The listing builds one solid part. Answer for the finished solid, in the listing's coordinates (mm). A direction names the side the tool comes from. Round coordinates to 2 decimals unless told otherwise and drop trailing zeros. Answer in a Markdown table with one row per item. Add a question column.
```python
from build123d import *

# Parameters (mm, degrees)
F1_DEPTH = 7
F2_R     = 2
F3_COUNT = 3


with BuildPart() as f1:
    # F0 (on Top) → F1 (new body)
    with BuildSketch(Plane.XY):
        with BuildLine():
            ThreePointArc((28, 0), (14, 14), (0, 0))
            Line((0, 0), (3.1437343742, 0))
            Line((3.1437343742, 0), (8.3414580162, 9.3975654268))
            Line((8.3414580162, 9.3975654268), (19.3092594014, 9.5992238198))
            Line((19.3092594014, 9.5992238198), (24.9678013852, 0.201658393))
            Line((24.9678013852, 0.201658393), (24.8562656258, 0))
            Line((24.8562656258, 0), (28, 0))
        make_face()
        with BuildLine():
            Line((3.1437343742, 0), (0, 0))
            ThreePointArc((0, 0), (14, -14), (28, 0))
            Line((28, 0), (24.8562656258, 0))
            Line((24.8562656258, 0), (19.6585419838, -9.3975654268))
            Line((19.6585419838, -9.3975654268), (8.6907405986, -9.5992238198))
            Line((8.6907405986, -9.5992238198), (3.0321986148, -0.201658393))
            Line((3.0321986148, -0.201658393), (3.1437343742, 0))
        make_face()
        with BuildLine():
            ThreePointArc((28, 0), (14, -14), (0, 0))
            Line((0, 0), (0, -30))
            ThreePointArc((0, -30), (14, -16), (28, -30))
            Line((28, -30), (28, 0))
        make_face()
        with BuildLine():
            Line((2.975, -30), (0, -30))
            ThreePointArc((0, -30), (14, -44), (28, -30))
            Line((28, -30), (25.025, -30))
            ThreePointArc((25.025, -30), (14, -41.025), (2.975, -30))
        make_face()
        with BuildLine():
            ThreePointArc((28, -30), (14, -16), (0, -30))
            Line((0, -30), (2.975, -30))
            ThreePointArc((2.975, -30), (14, -18.975), (25.025, -30))
            Line((25.025, -30), (28, -30))
        make_face()
    extrude(amount=F1_DEPTH)

    # F2
    f2_edges = [f1.edges().sort_by_distance(p)[0] for p in [
        (28, -15, 7),
        (14, 14, 7),
        (0, -15, 0),
        (14, -44, 0),
        (0, -15, 7),
        (14, -44, 7),
        (14, 14, 0),
        (28, -15, 0),
    ]]
    fillet(f2_edges, radius=F2_R)

    # F3: F1 ×3 about axis
    f3_axis = Axis((14, -30, 7), (0, 0, -1))


with BuildPart() as f1_1:
    add(f1.part)
    for i in range(1, F3_COUNT):
        add(f1.part.rotate(f3_axis, i * 360 / F3_COUNT))


solid = f1_1.part
```
Item 1: Flat-ended cylindrical pins translate along their axes: P1, Ø1, axis at x = 20, z = 5, coming from the +Y side; P2, Ø1, axis at x = 24.5, z = 4, coming from the -Y side; P3, Ø2.5, axis at y = -15.5, z = 3.5, coming from the -X side. Find the tip coordinate at first contact, or state that the pin passes through.
Item 2: For a pull along Y with two mould halves and no side action, classify faces 1 (the face through (-24.256, -51.732, 3.479)), 2 (the face through (12, -41, 0)), 3 (the face through (5.901, -4.966, 3.451)), 4 (the face through (-9.36, -27.32, 3.48)) as released by +Y, released by -Y, zero draft, split by the parting line, or undercut.
Item 3: The part is cut by section A-A, the plane z = 3.75. State how many separate pieces and enclosed holes the cut face has, and give its area (3 significant figures).
Item 4: Find the intervals of material crossed by probe 1 along Y at (x, z) = (16, 5.25); probe 2 along Y at (x, z) = (13.5, 5); probe 3 along X at (y, z) = (-49, 1.5), in increasing order. Write a range as [from, to].
Item 5: A tool of negligible diameter and unlimited length cuts with its end or side. For faces 5 (the face through (-3.9, -40, 3.5)), 6 (the face through (23.415, -50.943, 0.601)), 7 (the face through (23.415, -50.943, 6.399)), from which of +Z, -Z, +X, -X, +Y, -Y can it reach the whole face along a straight path? Write none if from no direction.
Resolved:
| question | item | result |
|---|---|---|
| 1 | P1 | y = 12.87 |
| 1 | P2 | y = -52.52 |
| 1 | P3 | x = 0 |
| 2 | face 1 | split by the parting line |
| 2 | face 2 | zero draft |
| 2 | face 3 | undercut |
| 2 | face 4 | released by +Y |
| 3 | separate pieces | 1 |
| 3 | enclosed holes | 4 |
| 3 | area | 1,780 mm2 |
| 4 | probe 1 | [-47.3, -40.84], [-19.16, -9.46], [9.54, 13.84] |
| 4 | probe 2 | [-46.45, -41.01], [-18.99, -9.51], [9.49, 13.99] |
| 4 | probe 3 | [-25.33, -20.66], [-3.34, 8.96], [19.04, 31.3], [48.62, 53.33] |
| 5 | face 5 | +Z, -Z |
| 5 | face 6 | -Z, -Y |
| 5 | face 7 | +Z, -Y |
